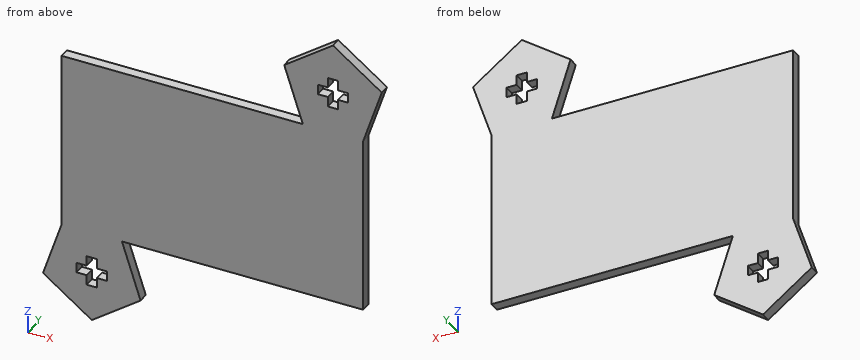
from build123d import *

# Parameters (mm, degrees)
BOSS_EXTRUDE1_DEPTH = 5.08


with BuildPart() as part:
    # Sketch1 → Boss-Extrude1 (new body)
    with BuildSketch(Plane(origin=(0, 0, 0), x_dir=(1, 0, 0), z_dir=(0, 1, 0))):
        Polygon((-74.783670705, 36.824993776), (-74.783670705, -53.334846224), (46.37500358, -53.334846224), (37.014119661, -82.142609318), (61.519803774, -99.947823692), (86.026241778, -82.14364696), (76.666369295, -53.334846224), (76.666369295, 36.824993776), (-44.491630705, 36.824993776), (-35.131758222, 65.633794512), (-59.638196226, 83.437971244), (-84.143880339, 65.63275687), align=None)
        Polygon((-59.637650705, 65.290773776), (-57.097650705, 65.290773776), (-57.097650705, 60.210773776), (-52.017650705, 60.210773776), (-52.017650705, 57.670773776), (-52.017650705, 55.130773776), (-57.097650705, 55.130773776), (-57.097650705, 50.050773776), (-59.637650705, 50.050773776), (-62.177650705, 50.050773776), (-62.177650705, 55.130773776), (-67.257650705, 55.130773776), (-67.257650705, 57.670773776), (-67.257650705, 60.210773776), (-62.177650705, 60.210773776), (-62.177650705, 65.290773776), align=None, mode=Mode.SUBTRACT)
        Polygon((69.140349295, -74.180626224), (69.140349295, -76.720626224), (64.060349295, -76.720626224), (64.060349295, -81.800626224), (61.520349295, -81.800626224), (58.980349295, -81.800626224), (58.980349295, -76.720626224), (53.900349295, -76.720626224), (53.900349295, -74.180626224), (53.900349295, -71.640626224), (58.980349295, -71.640626224), (58.980349295, -66.560626224), (61.520349295, -66.560626224), (64.060349295, -66.560626224), (64.060349295, -71.640626224), (69.140349295, -71.640626224), align=None, mode=Mode.SUBTRACT)
    extrude(amount=BOSS_EXTRUDE1_DEPTH)


solid = part.part
Geometry: final body of the model. Coordinates: model frame, mm. Give positions to 0.01 mm unless a question says otherwise; leave off trailing zeros. Loops run counter-clockwise (first coordinate to the right, second up) from the corner with the lowest first, then second, coordinate; pieces in that order, holes last. Notation, with made-up numbers: (63.5, 65) - (87.5, 65) arc R12 ccw to (87.5, 82) - close; hole circle Ø5 at (79, 69.25). An arc over 180 degrees is marked (long way). Answer as CSV lines item,"result". Start each with the question number.
1. Section B-B, the plane y = 2.1. Give the number of separate pieces and of enclosed holes in the cut face, plus the area to 3 significant figures.
2. Ray query, L1, parallel to Z at x = 7, y = 1.25 (3 decimals); L2, parallel to X at y = 0.8, z = -2; L3, parallel to X at y = 0.55, z = 74. Return the intervals inside material, ascending.
3. Section A-A, the plane x = 56. Return loops of the section in (y, z) (3 decimals), plus the area to 3 significant figures.
4. Pin query (flat end, axial travel): P1, Ø1.5, axis at y = 2.5, z = -62, coming from the -X side; P2, Ø3, axis at y = 4.5, z = -36.5, coming from the -X side; P3, Ø4, axis at x = 22.5, z = -38.5, coming from the +Y side; P4, Ø2.5, axis at x = -65.5, y = 1.5, coming from the -Z side. Return the tip coordinate at first contact, or that it passes through.
5. Section C-C, the plane z = 69. Return loops of the section in (x, y), plus the area to 3 significant figures.
6. Section D-D, the plane z = 41. Return loops of the section in (x, y).
Answers:
1,separate pieces,"1"
1,enclosed holes,"2"
1,area,"16,600 mm2"
2,L1,"z = -36.825 to 53.335"
2,L2,"x = -74.78 to 76.67"
2,L3,"x = 39.66 to 53.9, 69.14 to 83.38"
3,outline,"(0, -36.825) - (5.08, -36.825) - (5.08, 71.641) - (0, 71.641) - close; (0, 76.721) - (5.08, 76.721) - (5.08, 95.937) - (0, 95.937) - close"
3,area,"649 mm2"
4,P1,"stops at x = -83.21"
4,P2,"stops at x = -75.17"
4,P3,"stops at y = 5.08"
4,P4,"stops at z = -80.09"
5,outline,"(41.28, 0) - (58.98, 0) - (58.98, 5.08) - (41.28, 5.08) - close; (64.06, 0) - (81.76, 0) - (81.76, 5.08) - (64.06, 5.08) - close"
5,area,"180 mm2"
6,outline,"(-74.78, 0) - (76.67, 0) - (76.67, 5.08) - (-74.78, 5.08) - close"
